from build123d import *

# Parameters (mm, degrees)
SKETCH1_R           = 1
BOSS_EXTRUDE1_DEPTH = 2
SKETCH2_R           = 2
CUT_EXTRUDE1_DEPTH  = 1
BOSS_EXTRUDE2_DEPTH = 2
BOSS_EXTRUDE3_DEPTH = 1


with BuildPart() as part:
    # Sketch1 → Boss-Extrude1 (new body)
    with BuildSketch(Plane.XY):
        with BuildLine():
            Line((3, 0), (3, 3))
            Line((3, 3), (0, 3))
            ThreePointArc((0, 3), (-3, 0), (0, -3))
            Line((0, -3), (3, -3))
            Line((3, -3), (3, 0))
        make_face()
        Circle(SKETCH1_R, mode=Mode.SUBTRACT)
    extrude(amount=BOSS_EXTRUDE1_DEPTH)

    # Sketch2 → Cut-Extrude1 (cut)
    with BuildSketch(Plane.XY.offset(2)):
        Circle(SKETCH2_R)
    extrude(amount=-CUT_EXTRUDE1_DEPTH, mode=Mode.SUBTRACT)

    # Sketch3 → Boss-Extrude2 (add)
    with BuildSketch(Plane.XY.offset(2)):
        with BuildLine():
            Line((0, -2), (0, -3))
            Line((0, -3), (3, -3))
            Line((3, -3), (3, 0))
            Line((3, 0), (2, 0))
            ThreePointArc((2, 0), (1.414213562, -1.414213562), (0, -2))
        make_face()
    extrude(amount=BOSS_EXTRUDE2_DEPTH)

    # Sketch4 → Boss-Extrude3 (add)
    with BuildSketch(Plane.XY.offset(2)):
        with BuildLine():
            Line((-3, 0), (-2, 0))
            ThreePointArc((-2, 0), (-1.414213562, -1.414213562), (0, -2))
            Line((0, -2), (0, -3))
            ThreePointArc((0, -3), (-2.121320344, -2.121320344), (-3, 0))
        make_face()
    extrude(amount=BOSS_EXTRUDE3_DEPTH)


solid = part.part
Could you check a few things on this model? Use its own coordinates, in mm. A direction names the side the tool comes from. Give positions to 0.01 mm unless a question says otherwise; leave off trailing zeros. Order: outer loops, then holes, each group sorted by start corner. A loop starts at its lowest first (then second) coordinate and runs counter-clockwise, first axis right, second up.
1. I need wall thicknesses on L1, parallel to Y at x = 0, z = 0.5; L2, parallel to Z at x = 0.9, y = 0.55. Which ranges of each line are inside material? Lowest first, please.
2. Will these pins go through, and if not, where does the flat tip stop? P1, Ø0.5, axis at y = -2.5, z = 3.5, coming from the -X side; P2, Ø2.5, axis at x = 0, y = 0, coming from the +Z side; P3, Ø1.5, axis at x = -1, y = -1.5, coming from the +Z side.
3. For faces 4 (the flat face through (0, -2.5, 3.5)), 5 (the flat face through (1, -1, 1)), 6 (the flat face through (2.5, 0, 3)), which set-ups out of +Z, -Z, +X, -X, +Y, -Y let a thin tool reach every point of the face, with its end or its side?
4. We'd pull the mould along Y, two halves only. Please class faces 1 (the flat face through (1, 2, 2)), 2 (the cylindrical face through (-0.217, -0.976, 0.493)), 3 (the flat face through (-2.5, 0, 2.5)): pulls with the +Y half, pulls with the -Y half, needs draft (parallel to the pull), parting line crosses it, or undercut.
5. Suppose I cut it at A-A (x = 0.9). List the corners of the cut face in (y, z) for me, plus the area to 3 significant figures.
6. Suppose I cut it at B-B (z = 2.55). List the corners of the cut face in (x, y) for me.
7. Suppose I cut it at C-C (y = 0.85). List the corners of the cut face in (x, z) for me, plus the area to 3 significant figures.
8. Suppose I cut it at D-D (z = 1.2). List the corners of the cut face in (x, y) for me.
Solved:
1. L1: y = -3 to -1, 1 to 3
1. L2: z = 0 to 1
2. P1: stops at x = 0
2. P2: stops at z = 1
2. P3: stops at z = 3
3. face 4: +Z, -X, +Y, -Y
3. face 5: +Z
3. face 6: +Z, +X, -X, +Y
4. face 1: needs draft
4. face 2: undercut
4. face 3: pulls with the +Y half
5. outline: (-3, 0) - (-0.44, 0) - (-0.44, 1) - (-1.79, 1) - (-1.79, 4) - (-3, 4) - close; (0.44, 0) - (3, 0) - (3, 2) - (1.79, 2) - (1.79, 1) - (0.44, 1) - close
5. area: 9.98 mm2
6. outline: (-3, 0) arc R3 ccw to (0, -3) - (3, -3) - (3, 0) - (2, 0) arc R2 cw to (-2, 0) - close
7. outline: (-2.88, 0) - (-0.53, 0) - (-0.53, 1) - (-1.81, 1) - (-1.81, 2) - (-2.88, 2) - close; (0.53, 0) - (3, 0) - (3, 2) - (1.81, 2) - (1.81, 1) - (0.53, 1) - close
7. area: 7.08 mm2
8. outline: (0, -3) - (3, -3) - (3, 3) - (0, 3) arc R3 ccw to start; hole circle Ø4 at (0, 0)
